Autodesk Inventor part; units mm, degrees
ref_plane "YZ Plane" through (0, 0, 0) normal (1, 0, 0) x (0, 1, 0)
ref_plane "XZ Plane" through (0, 0, 0) normal (0, 1, 0) x (-1, 0, 0)
ref_plane "XY Plane" through (0, 0, 0) normal (0, 0, 1) x (1, 0, 0)
sketch "Sketch1" plane through (0, 0, 0) normal (0, 0, 1) x (1, 0, 0)
  line L0 (-2.2023, 4.6) -> (2.2023, 4.6)
  line L1 (-2.2023, -4.6) -> (2.2023, -4.6)
  line L2 (0, 0) -> (7.7204, 0) construction
  arc A0 (-2.2023, 4.6) -> (-2.2023, -4.6) centre (0, 0) ccw
  arc A1 (2.2023, -4.6) -> (2.2023, 4.6) centre (0, 0) ccw
  line L3 (0, 0) -> (-1, 0)
  circle A2 centre (-1, 0) radius 7
  line L4 (5.1, 0) -> (6, 0)
  dimension "d3" = 14
  dimension "d0" = 9.2
  dimension "d1" = 5.1
  dimension "d2" = 1
  dimension "d9" = 0.9
extrude "Extrusion1" add sketch "Sketch1" along normal blind 1
sketch "Sketch2" plane through (-1, 0, 1) normal (0, 0, 1) x (1, 0, 0)
  arc A0 (3.2023, -4.6) -> (3.2023, 4.6) centre (1, 0) ccw
  line L0 (3.2023, -4.6) -> (-1.2023, -4.6)
  arc A1 (-1.2023, 4.6) -> (-1.2023, -4.6) centre (1, 0) ccw
  line L1 (-1.2023, 4.6) -> (3.2023, 4.6)
  circle A2 centre (0, 0) radius 7
  circle A3 centre (1, 0) radius 6
  dimension "d6" = 12
extrude "Extrusion2" add sketch "Sketch2" along normal blind 1 contours A3
properties part number "top_clip" material "ABS Plastic"
Could you check a few things on this model? Use its own coordinates, in mm. A direction names the side the tool comes from. Give positions to 0.01 mm unless a question says otherwise; leave off trailing zeros. Order: outer loops, then holes, each group sorted by start corner. A loop starts at its lowest first (then second) coordinate and runs counter-clockwise, first axis right, second up.
Q1. If I drill on line 1 along X through (y, z) = (4.25, 1.7); line 2 along Y through (x, z) = (-1.5, 1.1); line 3 along Y through (x, z) = (1.75, 0.65), over which ranges is the centre line in solid material (lowest first)?
Q2. Suppose I cut it at D-D, the plane y = -5.5. Write out the boundary of the cut face in (x, z).
Q3. Suppose I cut it at A-A, the plane x = -1. Write out the boundary of the cut face in (y, z).
Q4. We'd pull the mould along Y, two halves only. Please class faces 1 (the flat face through (0, -4.6, 1)), 2 (the cylindrical face through (-5.994, -0.264, 1.493)), 3 (the flat face through (-6.2, 0.6, 1)): +Y half, -Y half, draft (parallel to the pull), parting line (faces both ways), or undercut.
Q5. Suppose I cut it at C-C, the plane y = 2.5. Write out the boundary of the cut face in (x, z), and give its area (3 significant figures).
Q6. Suppose I cut it at B-B, the plane z = 1.75. Write out the boundary of the cut face in (x, y).
Q7. For faces 4 (the cylindrical face through (5.1, 0.1, 1)), 5 (the flat face through (-4.2, 3.2, 0)), which set-ups out of +Z, -Z, +X, -X, +Y, -Y let a thin tool reach every point of the face, with its end or its side?
Solution:
1. line 1: x = -4.24 to -2.82, 2.82 to 4.24
1. line 2: y = -5.81 to -4.6, 4.6 to 5.81
1. line 3: y = -6.44 to -4.6, 4.6 to 6.44
2. outline: (-5.33, 0) - (3.33, 0) - (3.33, 1) - (2.4, 1) - (2.4, 2) - (-2.4, 2) - (-2.4, 1) - (-5.33, 1) - close
3. outline: (-7, 0) - (-4.6, 0) - (-4.6, 2) - (-5.92, 2) - (-5.92, 1) - (-7, 1) - close; (4.6, 0) - (7, 0) - (7, 1) - (5.92, 1) - (5.92, 2) - (4.6, 2) - close
4. face 1: undercut
4. face 2: parting line
4. face 3: draft
5. outline: (-7.54, 0) - (-4.45, 0) - (-4.45, 2) - (-5.45, 2) - (-5.45, 1) - (-7.54, 1) - close; (4.45, 0) - (5.54, 0) - (5.54, 1) - (5.45, 1) - (5.45, 2) - (4.45, 2) - close
5. area: 6.20 mm2
6. outline: circle Ø12 at (0, 0); hole (-2.2, -4.6) - (2.2, -4.6) arc R5.1 ccw to (2.2, 4.6) - (-2.2, 4.6) arc R5.1 ccw to start
7. face 4: +Z, -Z
7. face 5: -Z, +X, -X, +Y, -Y
